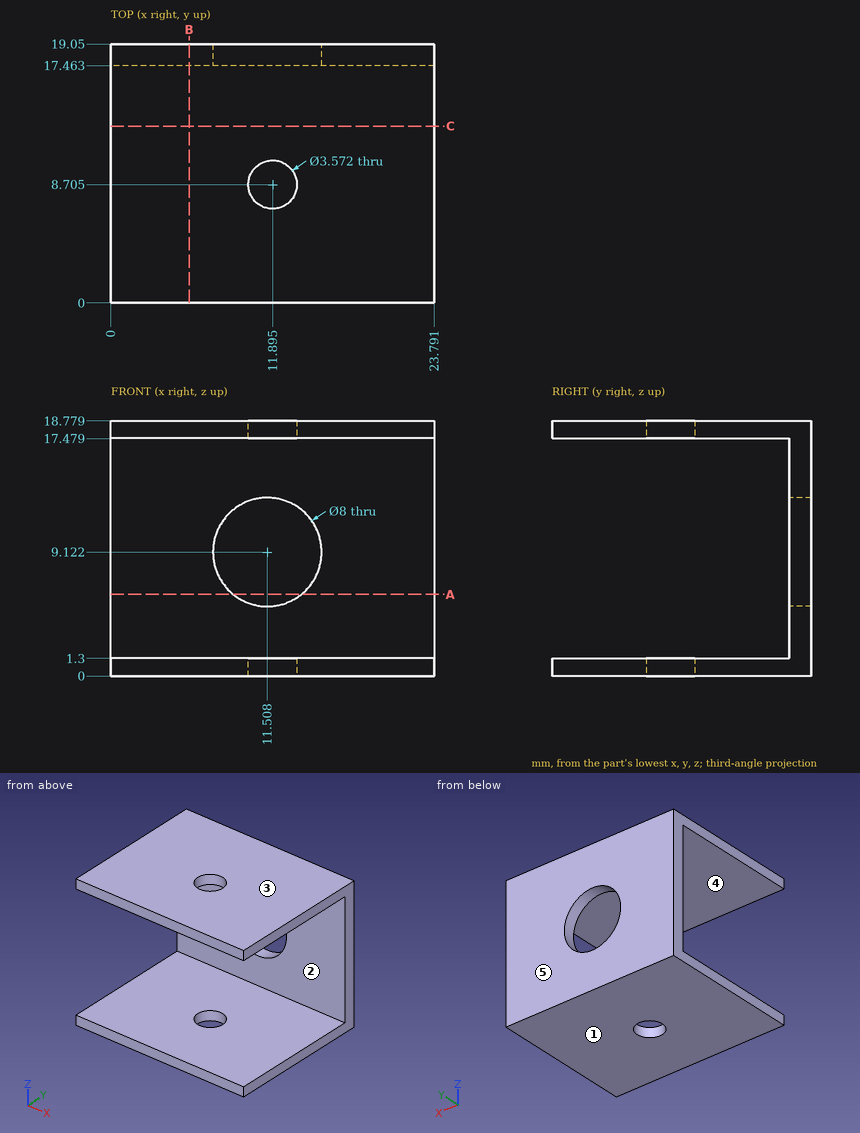
Input: dimensioned drawing with shaded views. Units: mm. Origin: part minimum x, y, z. A direction names the side the tool comes from. Coordinates: 2 decimals unless noted, no trailing zeros. Order: outer loops, then holes, each group sorted by start corner. A loop starts at its lowest first (then second) coordinate and runs counter-clockwise, first axis right, second up.
1. Cut plane B-B, the plane x = 5.75. Return loops of the section in (y, z).
Checked values:
outline: (0, 0) - (19.05, 0) - (19.05, 18.78) - (0, 18.78) - (0, 17.48) - (17.46, 17.48) - (17.46, 1.3) - (0, 1.3) - close
2. Ray query, line 1 along Z through (x, y) = (2, 13.5); line 2 along Y through (x, z) = (1.75, 6). Return the intervals inside material, ascending.
Checked values:
line 1: z = 0 to 1.3, 17.48 to 18.78
line 2: y = 17.46 to 19.05
3. Contact query for flat-ended pins moving along their axis: P1, Ø6, axis at x = 7, z = 4, coming from the -Y side; P2, Ø5, axis at x = 9.5, z = 7.5, coming from the -Y side. Output: stop coordinate, or through.
Checked values:
P1: stops at y = 0
P2: stops at y = 17.46
4. Access query for the marked faces 4 and 5. Directions: +Z, -Z, +X, -X, +Y, -Y. A direction counts if a zero-diameter tool reaches every point of the face in a straight line with its end or side. Return the directions, or none.
Checked values:
face 4: +X, -X, -Y
face 5: +Z, -Z, +X, -X, +Y
5. Cut plane C-C, the plane y = 13. Return loops of the section in (x, z).
Checked values:
outline: (0, 0) - (23.79, 0) - (23.79, 1.3) - (0, 1.3) - close; (0, 17.48) - (23.79, 17.48) - (23.79, 18.78) - (0, 18.78) - close
6. Cut plane A-A, the plane z = 6. Return loops of the section in (x, y).
Checked values:
outline: (0, 17.46) - (9.01, 17.46) - (9.01, 19.05) - (0, 19.05) - close; (14.01, 17.46) - (23.79, 17.46) - (23.79, 19.05) - (14.01, 19.05) - close
7. Draft query along Z for the marked faces 1, 2 and 3. Return one class per face: +Z half, -Z half, draft (parallel to the pull), parting line (faces both ways), or undercut.
Checked values:
face 1: -Z half
face 2: undercut
face 3: +Z half
